Autodesk Inventor part; units mm, degrees
ref_plane "YZ Plane" through (0, 0, 0) normal (1, 0, 0) x (0, 1, 0)
ref_plane "XZ Plane" through (0, 0, 0) normal (0, 1, 0) x (-1, 0, 0)
ref_plane "XY Plane" through (0, 0, 0) normal (0, 0, 1) x (1, 0, 0)
sketch "Sketch1" plane through (0, 0, 0) normal (0, 0, 1) x (1, 0, 0)
  line L0 (0, 0) -> (25.4, 0)
  line L1 (25.4, 0) -> (25.4, 25.4)
  line L2 (25.4, 25.4) -> (0, 25.4)
  line L3 (0, 25.4) -> (0, 0)
  line L4 (1.5875, 23.8125) -> (23.8125, 23.8125)
  line L5 (23.8125, 23.8125) -> (23.8125, 1.5875)
  line L6 (23.8125, 1.5875) -> (1.5875, 1.5875)
  line L7 (1.5875, 1.5875) -> (1.5875, 23.8125)
  dimension "d0" = 25.4
  dimension "d1" = 25.4
  dimension "d2" = 1.5875
extrude "Extrusion1" add sketch "Sketch1" against normal blind 355.6
sketch "Sketch2" plane through (0, 0, 0) normal (-1, 0, 0) x (0, 0, 1)
  line L0 (-355.6, 25.4) -> (-355.6, 0)
  line L1 (0, 0) -> (-355.6, 0)
  line L2 (0, 25.4) -> (0, 0)
  point P0 (-12.7, 12.7)
  point P1 (-342.9, 12.7)
  dimension "d5" = 12.7
  dimension "d6" = 12.7
  dimension "d7" = 12.7
hole "Hole1" at (0, 12.7, -12.7) at (0, 12.7, -342.9) direction (1, 0, 0) diameter 6.35 depth 25.4 tip angle 118
sketch "Sketch3" plane through (0, 25.4, 0) normal (0, 1, 0) x (1, 0, 0)
  line L0 (25.4, 355.6) -> (0, 355.6)
  line L1 (25.4, 0) -> (0, 0)
  point P0 (12.7, 12.7)
  point P1 (12.7, 342.9)
  dimension "d15" = 12.7
  dimension "d16" = 12.7
hole "Hole2" at (12.7, 25.4, -12.7) at (12.7, 25.4, -342.9) direction (0, -1, 0) diameter 6.35 depth 25.4 tip angle 118
properties part number "1tube_14_layer1_inside"
Check sheet for the modelled part. Datum: model origin and axes. Units: mm. A direction names the side the tool comes from. Coordinates: 2 decimals unless noted, no trailing zeros. Loops run counter-clockwise (first coordinate to the right, second up) from the corner with the lowest first, then second, coordinate; pieces in that order, holes last. Notation, with made-up numbers: (71, 79.25) -> (103, 79.25) arc R20 cw to (103, 90.25) -> close; hole circle Ø4 at (-28, 68.5). An arc over 180 degrees is marked (long way). Write item = value, one per line. Start each with the question number.
1. Section check A-A on y = 12.7. Record the cut outline in (x, z) (1 decimal).
2. Tool access check on faces 1 (the cylindrical face through (24.62, 11.75, -339.87)), 2 (the flat face through (13, 1.588, -175)). Record the directions out of +Z, -Z, +X, -X, +Y, -Y that give a thin tool (end or side, any length) a straight path to the whole face; none if there is none.
3. Section check C-C on z = -306.5. Record the cut outline in (x, y).
4. Depth check by flat-ended pin: P1, Ø3, axis at x = 5, z = -306.5, coming from the -Y side. Enter the tip coordinate at first touch or a pass-through.
5. Material ranges on line 1 (Z direction, x = 12.7, y = 0.7) (3 decimals); line 2 (Y direction, x = 0.4, z = -342.9) (3 decimals); line 3 (X direction, y = 23.75, z = -176), recorded low to high.
6. Draft check along Y on faces 3 (the cylindrical face through (15.5, 0.8, -11.2)), 4 (the flat face through (13, 0, -175)), 5 (the flat face through (13, 25.4, -175)), 6 (the flat face through (23.812, 13, -175)). Enter one of: released by +Y, released by -Y, zero draft, split by the parting line, or undercut.
Responses:
q1.outline = (0, -355.6) -> (1.6, -355.6) -> (1.6, -346.1) -> (0, -346.1) -> close; (0, -339.7) -> (1.6, -339.7) -> (1.6, -15.9) -> (0, -15.9) -> close; (0, -9.5) -> (1.6, -9.5) -> (1.6, 0) -> (0, 0) -> close; (23.8, -355.6) -> (25.4, -355.6) -> (25.4, -346.1) -> (23.8, -346.1) -> close; (23.8, -339.7) -> (25.4, -339.7) -> (25.4, -15.9) -> (23.8, -15.9) -> close; (23.8, -9.5) -> (25.4, -9.5) -> (25.4, 0) -> (23.8, 0) -> close
q2.face_1 = +X, -X
q2.face_2 = +Z, -Z
q3.outline = (0, 0) -> (25.4, 0) -> (25.4, 25.4) -> (0, 25.4) -> close; hole (1.59, 1.59) -> (23.81, 1.59) -> (23.81, 23.81) -> (1.59, 23.81) -> close
q4.P1 = 0
q5.line_1 = -355.6 to -346.075, -339.725 to -15.875, -9.525 to 0
q5.line_2 = 0 to 9.525, 15.875 to 25.4
q5.line_3 = 0 to 1.59, 23.81 to 25.4
q6.face_3 = zero draft
q6.face_4 = released by -Y
q6.face_5 = released by +Y
q6.face_6 = undercut
